```python
from build123d import *

# Parameters (mm, degrees)
CROQUIS1_W                       = 50
CROQUIS1_H                       = 20
CROQUIS1_R                       = 2.5
BRIDA_BASE1_DEPTH                = 3.03784
BRIDA_DE_ARISTA1_STRIP_W         = 18.50136
BRIDA_DE_ARISTA1_STRIP_H         = 3.03784
BRIDA_DE_ARISTA1_STRIP_CUT_DEPTH = 50
BRIDA_DE_ARISTA1_DEPTH           = 50
CORTAR_EXTRUIR1_REACH            = 58.837
CROQUIS9_R                       = 1.65


# Sheet-metal steps are written as plain solids
with BuildPart() as part:
    # Croquis1 → Brida base1 (new body)
    with BuildSketch(Plane.XY):
        Rectangle(CROQUIS1_W, CROQUIS1_H)
        with Locations((-12.7, 0)):
            Circle(CROQUIS1_R, mode=Mode.SUBTRACT)
        with Locations((12.7, 0)):
            Circle(CROQUIS1_R, mode=Mode.SUBTRACT)
    extrude(amount=-BRIDA_BASE1_DEPTH)

    # Brida de arista1 strip (across the edge) → Brida de arista1 strip cut (cut)
    with BuildSketch(Plane(origin=(-25, -10, 0), x_dir=(0, 1, 0), z_dir=(1, 0, 0))):
        with Locations((-3.03784, -1.51892)):
            Rectangle(BRIDA_DE_ARISTA1_STRIP_W, BRIDA_DE_ARISTA1_STRIP_H)
    extrude(amount=BRIDA_DE_ARISTA1_STRIP_CUT_DEPTH, mode=Mode.SUBTRACT)

    # Brida de arista1 section (across the edge) → Brida de arista1 (add)
    with BuildSketch(Plane(origin=(-25, -10, 0), x_dir=(0, 1, 0), z_dir=(1, 0, 0))):
        with BuildLine():
            Line((0, 3.175), (0, 46.96216))
            Line((0, 46.96216), (3.03784, 46.96216))
            Line((3.03784, 46.96216), (3.03784, 3.175))
            ThreePointArc((3.03784, 3.175), (3.96777597, 0.92993597), (6.21284, 0))
            Line((6.21284, 0), (6.21284, -3.03784))
            ThreePointArc((6.21284, -3.03784), (1.819698706, -1.218141294), (0, 3.175))
        make_face()
    extrude(amount=BRIDA_DE_ARISTA1_DEPTH)

    # Croquis9 → Cortar-Extruir1 (cut, up to next)
    with BuildSketch(Plane(origin=(0, -10, 0), x_dir=(-1, 0, 0), z_dir=(0, -1, 0)), mode=Mode.PRIVATE) as cortar_extruir1_sk1:
        with Locations(Location((0, -36.96216, 0), (0, 0, 90))):
            Circle(CROQUIS9_R)
    cortar_extruir1_tool1 = extrude(cortar_extruir1_sk1.sketch, amount=-CORTAR_EXTRUIR1_REACH, mode=Mode.PRIVATE) & part.part
    # Croquis9 → Cortar-Extruir1 (cut, up to next)
    with BuildSketch(Plane(origin=(0, -10, 0), x_dir=(-1, 0, 0), z_dir=(0, -1, 0)), mode=Mode.PRIVATE) as cortar_extruir1_sk2:
        with Locations(Location((0, -21.96216, 0), (0, 0, 90))):
            Circle(CROQUIS9_R)
    cortar_extruir1_tool2 = extrude(cortar_extruir1_sk2.sketch, amount=-CORTAR_EXTRUIR1_REACH, mode=Mode.PRIVATE) & part.part
    add(cortar_extruir1_tool1.solids().sort_by_distance((0, -10, 36.96216))[0], mode=Mode.SUBTRACT)
    add(cortar_extruir1_tool2.solids().sort_by_distance((0, -10, 21.96216))[0], mode=Mode.SUBTRACT)


solid = part.part
```
Input: part model. Units: mm. Frame: model coordinates. A direction names the side the tool comes from. Round coordinates to 2 decimals unless told otherwise and drop trailing zeros. Write each loop counter-clockwise with the first axis right and the second up, starting at its lowest first coordinate (ties: lowest second). Pieces come first, ordered by that corner, then holes. Notation, with made-up numbers: (-10.75, -1) - (35.25, -1) arc R7 cw to (35.25, 3) - close; hole circle Ø4 at (18.5, 64). An arc over 180 degrees is marked (long way). Write item = value, one per line.
(1) Section query D-D on z = 10.5. Output: boundary loops of the cut face in (x, y), then the cut area to 3 significant figures.
Geometry check:
outline = (-25, -10) - (25, -10) - (25, -6.96) - (-25, -6.96) - close
area = 152 mm^2
(2) Pull-direction query (X, two-part tool) for faces 1 (the cylindrical face through (0.07, -8.5, 38.61)), 2 (the flat face through (0, -9, 46.962)), 3 (the flat face through (25, -7.4, 14.7)); classes: +X half, -X half, draft (parallel to the pull), parting line (faces both ways), or undercut.
Geometry check:
face_1 = undercut
face_2 = draft
face_3 = +X half
(3) Section query C-C on x = -21.5. Output: boundary loops of the cut face in (y, z) (3 decimals).
Geometry check:
outline = (-10, 3.175) arc R6.213 ccw to (-3.787, -3.038) - (10, -3.038) - (10, 0) - (-3.787, 0) arc R3.175 cw to (-6.962, 3.175) - (-6.962, 46.962) - (-10, 46.962) - close
(4) Access query for faces 4 (the cylindrical face through (-15.2, 0.1, -1.5)), 5 (the flat face through (0, 3, 0)). Directions: +Z, -Z, +X, -X, +Y, -Y. A direction counts if a zero-diameter tool reaches every point of the face in a straight line with its end or side. Return the directions, or none.
Geometry check:
face_4 = +Z, -Z
face_5 = +Z, +X, -X, +Y
(5) Section query A-A on x = 12.7. Output: boundary loops of the cut face in (y, z) (3 decimals), then the cut area to 3 significant figures.
Geometry check:
outline = (-10, 3.175) arc R6.213 ccw to (-3.787, -3.038) - (-2.5, -3.038) - (-2.5, 0) - (-3.787, 0) arc R3.175 cw to (-6.962, 3.175) - (-6.962, 46.962) - (-10, 46.962) - close; (2.5, -3.038) - (10, -3.038) - (10, 0) - (2.5, 0) - close
area = 182 mm^2
(6) Section query B-B on x = 0. Output: boundary loops of the cut face in (y, z) (3 decimals), then the cut area to 3 significant figures.
Geometry check:
outline = (-10, 3.175) arc R6.213 ccw to (-3.787, -3.038) - (10, -3.038) - (10, 0) - (-3.787, 0) arc R3.175 cw to (-6.962, 3.175) - (-6.962, 20.312) - (-10, 20.312) - close; (-10, 23.612) - (-6.962, 23.612) - (-6.962, 35.312) - (-10, 35.312) - close; (-10, 38.612) - (-6.962, 38.612) - (-6.962, 46.962) - (-10, 46.962) - close
area = 177 mm^2
(7) Contact query for flat-ended pins moving along their axis: pin 1 Ø8 at (x, z) = (19, 36) entering from +Y; pin 2 Ø12 at (x, y) = (12.5, -1.5) entering from +Z; pin 3 Ø4 at (y, z) = (-4, 40) entering from -X; pin 4 Ø6.5 at (x, y) = (-12.7, 0) entering from +Z. Output: stop coordinate, or through.
Geometry check:
pin_1 = -6.96
pin_2 = 46.96
pin_3 = through
pin_4 = 0
(8) Material intervals for probe 1 along Y at (x, z) = (-20.5, 42.5); probe 2 along Y at (x, z) = (-12.7, -1.2); probe 3 along Y at (x, z) = (12, -1), sorted ascending.
Geometry check:
probe_1 = -10 to -6.96
probe_2 = -8.2 to -2.5, 2.5 to 10
probe_3 = -8.39 to -2.4, 2.4 to 10
